Design review of the part built by this model. Coordinates are the model's own, in mm. Face numbers are marked on the shaded views. A direction names the side the tool comes from. Give positions to 0.01 mm unless a question says otherwise; leave off trailing zeros. Loops run counter-clockwise (first coordinate to the right, second up) from the corner with the lowest first, then second, coordinate; pieces in that order, holes last. Notation, with made-up numbers: (-7.75, 7.5) -> (9.25, 7.5) arc R20 cw to (9.25, 21.5) -> close; hole circle Ø2 at (-7.75, 38.25). An arc over 180 degrees is marked (long way). Use CSV: the item, a comma, the result in double quotes. Start each with the question number.
Item 1: Wall thickness on line 1 along Y through (x, z) = (84, -51.5); line 2 along Z through (x, y) = (78.25, -8); line 3 along Z through (x, y) = (80.75, -10) (3 decimals): over which ranges is each line inside the solid? List them lowest first. Write a range as from..to.
Item 2: For the marked faces 1, 2, 3, 4 and 5, list the 3-axis set-ups (+Z, -Z, +X, -X, +Y, -Y) from which the entire face can be reached by the end or side of a thin tool; tool diameter is ignored.
Item 3: We need section B-B (x = 81.25). State the section outline as (y, z) points (3 decimals).
Item 4: The part is to be moulded in two halves that separate along Y. For the marked faces 6, 7 and 8, say which applies: +Y half, -Y half, draft (parallel to the pull), parting line (faces both ways), or undercut.
Item 5: Clearance check with flat-ended pins moving along their axes: pin 1 (5 mm diameter, centred on y = -22, z = -4.5, fed in from +X); pin 2 (1.5 mm diameter, centred on x = 80, z = -38, fed in from +Y). State where each tip first meets the part, or that it passes through.
Item 6: We need section A-A (z = -51.5). State the section outline as (x, y) points, plus the area to 3 significant figures.
Item 7: We need section D-D (y = -6.5). State the section outline as (x, z) points, plus the area to 3 significant figures.
Item 8: We need section C-C (y = 6). State the section outline as (x, z) points.
from build123d import *

# Parameters (mm, degrees)
SKETCH049_R         = 17
PAD030_DEPTH        = 10
SKETCH066_R         = 18.575
POCKET019_DEPTH     = 7
HOLE005_D           = 5.3
HOLE005_DEPTH       = 25
HOLE005_CBORE_D     = 8.7
HOLE005_CBORE_DEPTH = 5.4
SKETCH061_R         = 2.2
POCKET021_DEPTH     = 10.001


with BuildPart() as part:
    # Sketch049 → Pad030 (new body)
    with BuildSketch(Plane.YZ.offset(81)):
        with BuildLine():
            ThreePointArc((1, -34.657656), (6.482261, 11.385394), (-36.646111, -5.64285))
            Line((-43, -44.5), (-36.646111, -5.64285))
            Line((-43, -58.5), (-43, -44.5))
            Line((-43, -58.5), (1, -58.5))
            Line((1, -58.5), (1, -34.657656))
        make_face()
        with Locations((-10, -10)):
            Circle(SKETCH049_R, mode=Mode.SUBTRACT)
    extrude(amount=PAD030_DEPTH)

    # Sketch066 → Pocket019 (cut)
    with BuildSketch(Plane.YZ.offset(91)):
        with Locations((-10, -10)):
            Circle(SKETCH066_R)
    extrude(amount=-POCKET019_DEPTH, mode=Mode.SUBTRACT)

    # Hole005
    with Locations(Plane(origin=(81, 0, 0), x_dir=(0, 1, 0), z_dir=(-1, 0, 0))):
        with Locations((-34, 51.5), (-8, 51.5)):
            CounterBoreHole(HOLE005_D / 2, HOLE005_CBORE_D / 2, HOLE005_CBORE_DEPTH, depth=HOLE005_DEPTH)

    # Sketch061 → Pocket021 (cut, through all)
    with BuildSketch(Plane.YZ.offset(81)):
        with Locations((-29.052559, 1)):
            Circle(SKETCH061_R)
        with Locations((9.052559, 1)):
            Circle(SKETCH061_R)
        with Locations((-10, -32)):
            Circle(SKETCH061_R)
    extrude(amount=POCKET021_DEPTH, mode=Mode.SUBTRACT)


with BuildPart() as part_1:
    # Body012 placement: moved
    add(part.part.moved(Location((-6, 0, 0))))


solid = part_1.part
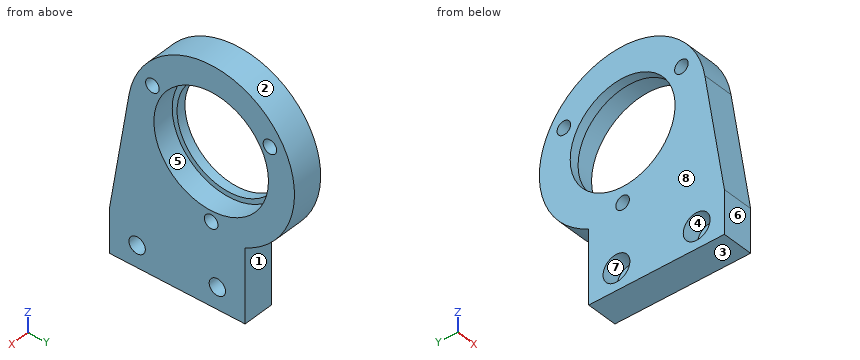
Results found:
1,line 1,"-43..-36.65, -31.35..-10.65, -5.35..1"
1,line 2,"-58.5..-55.85, -47.15..-32.92, -31.08..-28.47, 8.47..16.93"
1,line 3,"-58.5..-53.239, -49.761..-34.2, -29.8..-28.575, 8.575..17"
2,face 1,"-Z, +X, -X, +Y"
2,face 2,"+X, -X"
2,face 3,"-Z, +X, -X, +Y, -Y"
2,face 4,"-X"
2,face 5,"+X"
3,outline,"(-43, -58.5) -> (1, -58.5) -> (1, -34.658) arc R27 ccw (long way) to (-36.646, -5.643) -> (-43, -44.5) -> close; hole circle Ø5.3 at (-34, -51.5); hole circle Ø4.4 at (-29.053, 1); hole circle Ø37.15 at (-10, -10); hole circle Ø4.4 at (-10, -32); hole circle Ø5.3 at (-8, -51.5); hole circle Ø4.4 at (9.053, 1)"
4,face 6,"-Y half"
4,face 7,"undercut"
4,face 8,"draft"
5,pin 1,"through"
5,pin 2,"y = 1"
6,outline,"(75, -43) -> (85, -43) -> (85, -36.65) -> (80.4, -36.65) -> (80.4, -38.35) -> (75, -38.35) -> close; (75, -29.65) -> (80.4, -29.65) -> (80.4, -31.35) -> (85, -31.35) -> (85, -10.65) -> (80.4, -10.65) -> (80.4, -12.35) -> (75, -12.35) -> close; (75, -3.65) -> (80.4, -3.65) -> (80.4, -5.35) -> (85, -5.35) -> (85, 1) -> (75, 1) -> close"
6,area,"297 mm²"
7,outline,"(75, -58.5) -> (85, -58.5) -> (85, -53.68) -> (80.4, -53.68) -> (80.4, -55.58) -> (75, -55.58) -> close; (75, -47.42) -> (80.4, -47.42) -> (80.4, -49.32) -> (85, -49.32) -> (85, -28.24) -> (78, -28.24) -> (78, -26.64) -> (75, -26.64) -> close; (75, 6.64) -> (78, 6.64) -> (78, 8.24) -> (85, 8.24) -> (85, 16.77) -> (75, 16.77) -> close"
7,area,"333 mm²"
8,outline,"(75, -31.75) -> (85, -31.75) -> (85, -19.44) -> (78, -19.44) -> (78, -15.74) -> (75, -15.74) -> close; (75, -4.26) -> (78, -4.26) -> (78, -0.56) -> (85, -0.56) -> (85, 11.75) -> (75, 11.75) -> close"
